Read the model definition and answer for the solid it produces. Units are mm, in the model's axes. A direction names the side the tool comes from. Give positions to 0.01 mm unless a question says otherwise; leave off trailing zeros. Write each loop counter-clockwise with the first axis right and the second up, starting at its lowest first coordinate (ties: lowest second). Pieces come first, ordered by that corner, then holes. Notation, with made-up numbers: (20.25, 47.5) - (36.25, 47.5) arc R18 ccw to (36.25, 66.5) - close; hole circle Ø5 at (31, -8). An arc over 180 degrees is marked (long way). Answer as CSV lines item,"result".
Autodesk Inventor part; units mm, degrees
ref_plane "YZ Plane" through (0, 0, 0) normal (1, 0, 0) x (0, 1, 0)
ref_plane "XZ Plane" through (0, 0, 0) normal (0, 1, 0) x (-1, 0, 0)
ref_plane "XY Plane" through (0, 0, 0) normal (0, 0, 1) x (1, 0, 0)
sketch "Sketch1" plane through (0, 0, 0) normal (0, 0, 1) x (1, 0, 0)
  line L0 (0, 0) -> (10, 0)
  line L1 (10, 0) -> (10, 9)
  line L2 (10, 9) -> (0, 9)
  line L3 (0, 9) -> (0, 0)
  point P0 (5, 9)
  dimension "d0" = 10
  dimension "d1" = 9
extrude "Extrusion1" add sketch "Sketch1" along normal blind 3
sketch "Sketch2" plane through (0, 0, 3) normal (0, 0, 1) x (1, 0, 0)
  line L0 (10, 9) -> (0, 9)
  circle A0 centre (5, 7) radius 1
  line L1 (0, 9) -> (0, 0)
  point P0 (5, 9)
  dimension "d4" = 2
  dimension "d5" = 2
  dimension "d67" = 5
extrude "Extrusion2" add sketch "Sketch2" along normal blind 1.5
sketch "Sketch6" plane through (5, 7, 4.5) normal (0, 0, 1) x (1, 0, 0)
  circle A0 centre (0, 0) radius 1
  line L0 (2, -1) -> (-2, -1)
  line L1 (-2, -1) -> (-2, 1)
  line L2 (-2, 1) -> (2, 1)
  line L3 (2, 1) -> (2, -1)
  line L4 (2, -1) -> (-2, 1) construction
  line L5 (-2, -1) -> (2, 1) construction
  point P0 (-5, -7)
  dimension "d13" = 4
extrude "Extrusion5" add sketch "Sketch6" along normal blind 25
sketch "Sketch7" plane through (5, 7, 29.5) normal (0, 0, 1) x (1, 0, 0)
  circle A0 centre (0, 0) radius 1
  line L0 (-5, -7) -> (5, -7)
  line L1 (5, -7) -> (5, 2)
  line L2 (5, 2) -> (-5, 2)
  line L3 (-5, 2) -> (-5, -7)
  arc A1 (0, -1) -> (0, 1) centre (0, 0) ccw
  arc A2 (0, 1) -> (0, -1) centre (0, 0) ccw
extrude "Extrusion6" add sketch "Sketch7" along normal blind 4 contours A0 | L3 L2 L1 L0
sketch "Sketch8" plane through (5, 7, 33.5) normal (0, 0, 1) x (1, 0, 0)
  line L0 (-5, -7) -> (5, -7)
  line L1 (5, -7) -> (5, 2)
  line L2 (5, 2) -> (-5, 2)
  line L3 (-5, 2) -> (-5, -7)
  circle A0 centre (0, -3.5) radius 1.65
  dimension "d18" = 3.3
  dimension "d66" = 5.5
extrude "Extrusion7" cut sketch "Sketch8" against normal blind 4 contours A0
sketch "Sketch10" plane through (0, 0, 0) normal (-1, 0, 0) x (0, 0, 1)
  line L0 (0, 0) -> (3, 0)
  line L1 (3, 0) -> (2.5, 0)
  line L2 (2.5, 0) -> (2.5, 0.5)
  line L3 (2.5, 6) -> (3, 6)
  line L4 (3, 6) -> (3, 5)
  line L5 (3, 0) -> (2.5, 0.5)
  line L6 (3, 0) -> (3.7071, 0) construction
  line L7 (2.5, 0.5) -> (3, 1)
  line L8 (3, 1) -> (2.5, 1.5)
  line L9 (2.5, 1.5) -> (3, 2)
  line L10 (3, 2) -> (2.5, 2.5)
  line L11 (2.5, 2.5) -> (3, 3)
  line L12 (3, 3) -> (2.5, 3.5)
  line L13 (2.5, 3.5) -> (3, 4)
  line L14 (3, 4) -> (2.5, 4.5)
  line L15 (2.5, 4.5) -> (3, 5)
  line L16 (3, 5) -> (2.5, 5.5)
  line L17 (2.5, 5.5) -> (3, 6)
  line L18 (2.5, 5.5) -> (2.5, 6)
  line L19 (2.5, 4.5) -> (2.5, 5.5)
  line L20 (2.5, 3.5) -> (2.5, 4.5)
  line L21 (2.5, 2.5) -> (2.5, 3.5)
  line L22 (2.5, 1.5) -> (2.5, 2.5)
  line L23 (2.5, 0.5) -> (2.5, 1.5)
  line L24 (3, 1) -> (3, 0)
  line L25 (3, 2) -> (3, 1)
  line L26 (3, 3) -> (3, 2)
  line L27 (3, 5) -> (3, 4)
  line L28 (3, 4) -> (3, 3)
  point P0 (2.5, 3)
  point P1 (3, 4.4114)
  point P2 (2.5, 4.5886)
  dimension "d23" = 0.5
  dimension "d24" = 6
  dimension "d25" = 135
extrude "Extrusion10" add sketch "Sketch6" against normal up to surface (1.5 mm away) contours A0 L2 L3 L0 | A0 L0 L1 L2
sketch "Sketch12" plane through (5, 7, 29.5) normal (0, 0, -1) x (-1, 0, 0)
  circle A0 centre (0, 0) radius 1
  line L0 (-2, 1) -> (-2, -1)
  line L1 (-2, -1) -> (2, -1)
  line L2 (2, 1) -> (-2, 1)
  line L3 (2, -1) -> (2, 1)
  point P0 (5, -7)
extrude "Extrusion11" cut sketch "Sketch12" along normal blind 4 contours A0 L2 L3 L1 | A0 L1 L0 L2
chamfer "Chamfer3" distance 2 distance2 1 1 edges at (3, 7, 25.5) measured on face at (3, 6.6667, 10.5)
chamfer "Chamfer4" distance 2 distance2 1 1 edges at (7, 7, 25.5) measured on face at (7, 7.3333, 10.5)
extrude "Extrusion12" cut sketch "Sketch10" against normal up to next contours L5 L7 L24 | L8 L9 L25 | L10 L11 L26 | L12 L13 L28 | L14 L15 L27 | L16 L17 L4 | L18 L3 L17
properties part number "gravity-clamp-base5x5mm-part1-narrowTOP"
(1) A cutting plane is placed at A-A (x = 2.25). Write down the section's boundary in (y, z).
Worked out:
outline,"(0, 0) - (9, 0) - (9, 3) - (6, 3) - (6, 2.5) - (5.5, 2.5) - (5, 3) - (4.5, 2.5) - (4, 3) - (3.5, 2.5) - (3, 3) - (2.5, 2.5) - (2, 3) - (1.5, 2.5) - (1, 3) - (0.5, 2.5) - (0, 3) - close; (0, 29.5) - (9, 29.5) - (9, 33.5) - (0, 33.5) - close"
(2) For faces 4 (the flat face through (4.9, 8.2, 3)), 5 (the flat face through (3.5, 7, 24.5)), 6 (the flat face through (7, 7, 13)), 7 (the cylindrical face through (4.324, 6.263, 27.528)), determine the directions among +Z, -Z, +X, -X, +Y, -Y from which every point of the face is accessible in a straight line to the end or side of a thin tool.
Worked out:
face 4,"+Y"
face 5,"-X, +Y, -Y"
face 6,"+X, +Y, -Y"
face 7,"none"
(3) Find the intervals of material crossed by L1, parallel to Y at x = 5, z = 31.35; L2, parallel to Z at x = 9.25, y = 7.5; L3, parallel to Z at x = 7, y = 4.75, in increasing order.
Worked out:
L1,"y = 0 to 1.85, 5.15 to 9"
L2,"z = 0 to 3, 29.5 to 33.5"
L3,"z = 0 to 2.75, 29.5 to 33.5"
(4) Each of these flat-tipped pins is pushed along its axis until it touches: P1, Ø3, axis at x = 4, z = 19, coming from the -Y side; P2, Ø1.5, axis at y = 8, z = 27, coming from the +X side; P3, Ø5, axis at x = 2.5, z = 9.5, coming from the +Y side. Where does it stop, or does it pass through?
Worked out:
P1,"stops at y = 6"
P2,"stops at x = 5.97"
P3,"stops at y = 8"
(5) A cutting plane is placed at C-C (z = 4.5). Write down the section's boundary in (x, y).
Worked out:
outline,"(3, 6) - (7, 6) - (7, 8) - (3, 8) - close"
(6) The mould has two halves that part along Z. Classify faces 1 (the flat face through (3, 7, 13)), 2 (the flat face through (5, 0, 1)), 3 (the flat face through (5, 5, 0)): +Z half, -Z half, draft (parallel to the pull), parting line (faces both ways), or undercut.
Worked out:
face 1,"undercut"
face 2,"draft"
face 3,"-Z half"
